Geometry: final body of the model. Coordinates: model frame, mm. Coordinates: 2 decimals unless noted, no trailing zeros. Order: outer loops, then holes, each group sorted by start corner. A loop starts at its lowest first (then second) coordinate and runs counter-clockwise, first axis right, second up. Notation, with made-up numbers: M 1,-9 L 43,-9 A19 ccw 43,23 Z; hole C -15.75,43.5 d5. An arc over 180 degrees is marked long. Use CSV: the item, a comma, the result in double quotes. Start each with the question number.
Q1. Section query C-C, the plane y = 186.5. Output: boundary loops of the cut face in (x, z), and give its area (3 significant figures).
Q2. Section query D-D, the plane z = 9. Output: boundary loops of the cut face in (x, y).
Q3. Section query B-B, the plane z = 84. Output: boundary loops of the cut face in (x, y), and give its area (3 significant figures).
Q4. Ray query, probe 1 along Z at (x, y) = (6.75, 225); probe 2 along Y at (x, z) = (6.5, 63.5); probe 3 along Z at (x, y) = (5, 5.5). Return the intervals inside material, ascending.
Q5. First-contact query: P1, Ø5, axis at x = 5, z = 56.06, coming from the -Y side; P2, Ø3.5, axis at x = 5, z = 74.06, coming from the +Y side; P3, Ø12, axis at y = 61, z = 40.5, coming from the +X side; P4, Ø3, axis at x = 7, z = 59, coming from the +Y side. Flat tips, straight axial feed; report the tip coordinate or a pass-through.
Q6. Section query A-A, the plane y = 25.5. Output: boundary loops of the cut face in (x, z), and give its area (3 significant figures).
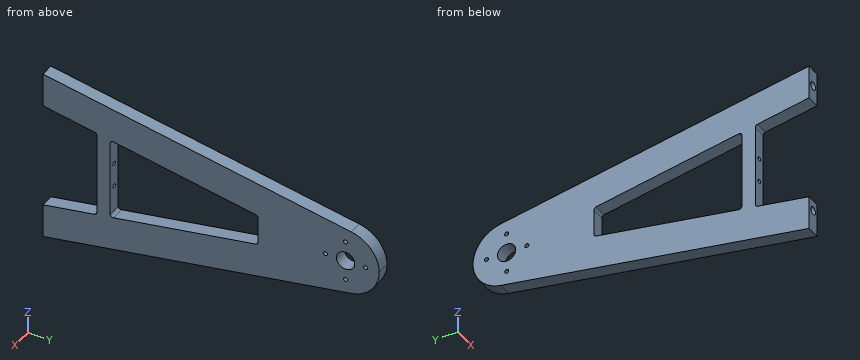
Autodesk Inventor part; units mm, degrees
ref_plane "YZ Plane" through (0, 0, 0) normal (1, 0, 0) x (0, 1, 0)
ref_plane "XZ Plane" through (0, 0, 0) normal (0, 1, 0) x (-1, 0, 0)
ref_plane "XY Plane" through (0, 0, 0) normal (0, 0, 1) x (1, 0, 0)
sketch "Skizze1" plane through (0, 0, 0) normal (1, 0, 0) x (0, 1, 0)
  arc A0 (250, 65.0592) -> (229.3412, 89.6794) centre (225, 65.0592) ccw
  line L0 (225, 65.0592) -> (229.3412, 89.6794) construction
  line L1 (225, 65.0592) -> (250, 65.0592) construction
  line L2 (229.3412, 89.6794) -> (0, 130.1185)
  line L3 (0, 130.1185) -> (0, 104.7328)
  arc A1 (229.3412, 40.439) -> (250, 65.0592) centre (225, 65.0592) ccw
  line L4 (229.3412, 40.439) -> (0, 0)
  line L5 (0, 0) -> (92.864, 0) construction
  line L6 (0, 0) -> (0, 25.3857)
  line L7 (160, 76.5205) -> (160, 53.598)
  line L8 (40, 97.6797) -> (40, 32.4387)
  line L9 (50, 34.202) -> (50, 95.9165)
  line L10 (0, 104.7328) -> (40, 97.6797)
  line L11 (50, 95.9165) -> (160, 76.5205)
  line L12 (0, 25.3857) -> (40, 32.4387)
  line L13 (50, 34.202) -> (160, 53.598)
  dimension "d21" = 80
  dimension "d24" = 25
  dimension "d68" = 250
  dimension "d73" = 80
  dimension "d88" = 130.1185
  dimension "d89" = 79.3471
  dimension "d91" = 10
  dimension "d92" = 25
  dimension "d93" = 25
  dimension "d94" = 40
  dimension "d96" = 25
  dimension "d97" = 25
  dimension "d127" = 110
extrude "Extrusion2" add sketch "Skizze1" along normal blind 10
sketch "Skizze7" plane through (10, 0, 0) normal (1, 0, 0) x (0, 0, -1)
  arc A0 (-40.439, 229.3412) -> (-89.6794, 229.3412) centre (-65.0592, 225) ccw
  point P0 (0, 0)
hole "Bohrung6" at (10, 225, 65.0592) direction (-1, 0, 0) diameter 13.6 end through all
sketch "Skizze8" plane through (10, 0, 0) normal (1, 0, 0) x (0, 0, -1)
  circle A0 centre (-65.0592, 225) radius 6.8
  line L0 (-65.0592, 225) -> (-65.0592, 240) construction
  point P0 (0, 0)
  point P1 (-80.0592, 225)
  point P2 (-65.0592, 210)
  point P3 (-50.0592, 225)
  dimension "d107" = 15
  dimension "d110" = 360
hole "Bohrung7" at (10, 240, 65.0592) at (10, 225, 80.0592) at (10, 210, 65.0592) at (10, 225, 50.0592) direction (-1, 0, 0) diameter 3 end through all
sketch "Skizze9" plane through (0, 0, 104.7328) normal (0, -1, 0) x (1, 0, 0)
  line L0 (0, 25.3857) -> (10, 25.3857) construction
  line L1 (5, 25.3857) -> (5, -104.7328) construction
  line L2 (0, -104.7328) -> (10, -104.7328) construction
  line L3 (0, 25.3857) -> (0, 0) construction
  line L4 (10, 25.3857) -> (10, 0) construction
  line L5 (0, 25.3857) -> (0, 0) construction
  line L6 (0, 0) -> (10, 0) construction
  line L7 (10, 25.3857) -> (10, 0) construction
  line L8 (0, 25.3857) -> (10, 25.3857) construction
  line L9 (0, 12.6928) -> (10, 12.6928) construction
  point P0 (5, 12.6928)
  point P1 (5, -87.3072)
  dimension "d119" = 100
hole "Bohrung8" at (5, 0, 117.4256) at (5, 0, 17.4256) direction (0, 1, 0) diameter 6 depth 20 tip angle 118
sketch "Skizze10" plane through (0, 50, 95.9165) normal (0, 1, 0) x (1, 0, 0)
  line L0 (10, 61.7144) -> (10, 0) construction
  line L1 (10, 30.8572) -> (0, 30.8572) construction
  point P0 (0, 95.9165)
  point P1 (5, 21.8572)
  point P2 (5, 39.8572)
  dimension "d128" = 5
  dimension "d130" = 9
  dimension "d132" = 5
  dimension "d133" = 18
hole "Bohrung9" at (5, 50, 74.0592) at (5, 50, 56.0592) direction (0, -1, 0) diameter 3 end through all
fillet "Rundung1" radius 2 6 edges at (5, 160, 76.5205) (5, 40, 97.6797) (5, 50, 95.9165) (5, 50, 34.202) (5, 160, 53.598) (5, 40, 32.4387)
properties part number "halter_seite"
Responses:
1,outline,"M 0,32.88 L 10,32.88 L 10,97.23 L 0,97.23 Z"
1,area,"643 mm²"
2,outline,"M 0,0 L 10,0 L 10,51.04 L 0,51.04 Z"
3,outline,"M 0,40 L 10,40 L 10,50 L 0,50 Z; M 0,117.58 L 10,117.58 L 10,241.32 L 0,241.32 Z"
3,area,"1,340 mm²"
4,probe 1,"z = 39.67 to 48.56, 51.56 to 58.26, 71.86 to 78.56, 81.56 to 90.44"
4,probe 2,"y = 40 to 50, 160 to 218.38, 231.62 to 249.95"
4,probe 3,"z = 0.97 to 14.43, 20.43 to 26.36, 103.76 to 114.43, 120.43 to 129.15"
5,P1,"stops at y = 40"
5,P2,"stops at y = 248.93"
5,P3,"stops at x = 10"
5,P4,"stops at y = 249.58"
6,outline,"M 0,4.5 L 10,4.5 L 10,29.88 L 0,29.88 Z; M 0,100.24 L 10,100.24 L 10,125.62 L 0,125.62 Z"
6,area,"508 mm²"
